Model file for the job. Use its own axes, mm. Round coordinates to 2 decimals unless told otherwise and drop trailing zeros. Loops run counter-clockwise (first coordinate to the right, second up) from the corner with the lowest first, then second, coordinate; pieces in that order, holes last. Notation, with made-up numbers: (54, 43.5) -> (77, 43.5) arc R24 cw to (77, 70.5) -> close; hole circle Ø2 at (34, -8.5). An arc over 180 degrees is marked (long way). Use a Markdown table: item, result. Add a question column.
```python
from build123d import *

# Parameters (mm, degrees)
BOSS_EXTRUDE1_DEPTH = 50.8


with BuildPart() as part:
    # Sketch1 → Boss-Extrude1 (new body)
    with BuildSketch(Plane.XY):
        with BuildLine():
            ThreePointArc((25.4, 50.8), (12.7, 63.5), (0, 50.8))
            Line((0, 50.8), (9.525, 50.8))
            ThreePointArc((9.525, 50.8), (12.7, 53.975), (15.875, 50.8))
            Line((15.875, 50.8), (25.4, 50.8))
        make_face()
        with BuildLine():
            Line((9.525, 50.8), (0, 50.8))
            ThreePointArc((0, 50.8), (12.7, 38.1), (25.4, 50.8))
            Line((25.4, 50.8), (15.875, 50.8))
            ThreePointArc((15.875, 50.8), (12.7, 47.625), (9.525, 50.8))
        make_face()
        with BuildLine():
            Line((0, 50.8), (0, 0))
            Line((0, 0), (25.4, 0))
            Line((25.4, 0), (25.4, 50.8))
            ThreePointArc((25.4, 50.8), (12.7, 38.1), (0, 50.8))
        make_face()
    extrude(amount=BOSS_EXTRUDE1_DEPTH)


solid = part.part
```
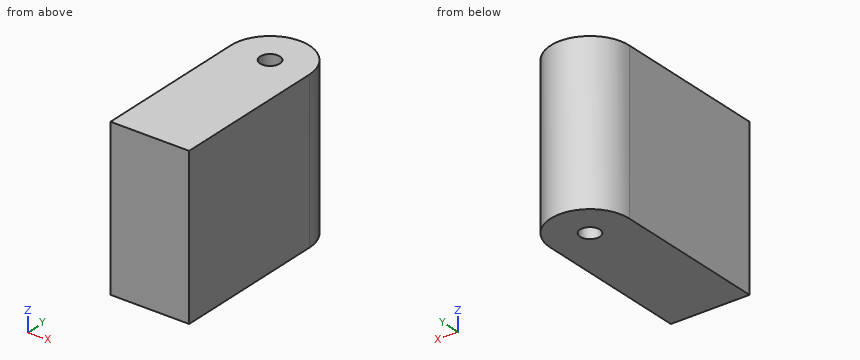
1) Cut at A-A on x = 12.7. Write the cut outline in (y, z) (3 decimals), and give its area (3 significant figures).
2) Pin check, flat tip, straight feed: pin 1 Ø6 at (x, z) = (19.5, 27.5) entering from +Y. Stop position of the tip, or through.
3) Wall check: probe 1 along X at (y, z) = (50.8, 22.5) (3 decimals); probe 2 along Y at (x, z) = (12.7, 35) (3 decimals); probe 3 along Y at (x, z) = (14.5, 39). Give the ranges that are in metal, low to high. Write a range as from..to.
4) Cut at C-C on x = 21.5. Write the cut outline in (y, z), and give its area (3 significant figures).
5) Cut at B-B on z = 47. Write the cut outline in (x, y) (3 decimals).
Established:
| question | item | result |
|---|---|---|
| 1 | outline | (0, 0) -> (47.625, 0) -> (47.625, 50.8) -> (0, 50.8) -> close; (53.975, 0) -> (63.5, 0) -> (63.5, 50.8) -> (53.975, 50.8) -> close |
| 1 | area | 2,900 mm^2 |
| 2 | pin 1 | stops at y = 62.92 |
| 3 | probe 1 | x = 0..9.525, 15.875..25.4 |
| 3 | probe 2 | y = 0..47.625, 53.975..63.5 |
| 3 | probe 3 | y = 0..48.18, 53.42..63.37 |
| 4 | outline | (0, 0) -> (59.96, 0) -> (59.96, 50.8) -> (0, 50.8) -> close |
| 4 | area | 3,050 mm^2 |
| 5 | outline | (0, 0) -> (25.4, 0) -> (25.4, 50.8) arc R12.7 ccw to (0, 50.8) -> close; hole circle Ø6.35 at (12.7, 50.8) |
